The model under review builds one solid part; all positions refer to its coordinate system, in mm. A direction names the side the tool comes from. Give positions to 0.01 mm unless a question says otherwise; leave off trailing zeros. Loops run counter-clockwise (first coordinate to the right, second up) from the corner with the lowest first, then second, coordinate; pieces in that order, holes last. Notation, with made-up numbers: (-6, 11.25) - (10, 11.25) arc R20 cw to (10, 33.25) - close; hole circle Ø8 at (70.25, 88). An arc over 180 degrees is marked (long way). Return JSON: item names as keys, results as strings. Group by question number.
from build123d import *

# Parameters (mm, degrees)
SKETCH1_R               = 18
BOSS_EXTRUDE1_DEPTH     = 70
SKETCH2_R               = 2.5
BOSS_EXTRUDE2_DEPTH     = 17
CUT_EXTRUDE1_START      = -15
CUT_EXTRUDE1_DEPTH      = 15
SKETCH4_R               = 1.5875
CUT_EXTRUDE2_DEPTH      = 12.7
CIRPATTERN1_COUNT       = 6
BOSS_EXTRUDE3_START     = -2.032
BOSS_EXTRUDE3_DEPTH     = 8.382
BOSS_EXTRUDE4_DEPTH     = 12.0015
CUT_EXTRUDE3_REACH      = 99.88
CUT_EXTRUDE3_END_RADIUS = 18.8128
SKETCH7_R               = 2.159


with BuildPart() as part:
    # Sketch1 → Boss-Extrude1 (new body)
    with BuildSketch(Plane(origin=(0, 0, 0), x_dir=(1, 0, 0), z_dir=(0, 1, 0))):
        with Locations(Location((0, 0, 0), (0, 0, 270))):
            Circle(SKETCH1_R)
    extrude(amount=BOSS_EXTRUDE1_DEPTH)

    # Sketch2 → Boss-Extrude2 (add)
    with BuildSketch(Plane(origin=(0, 70, 0), x_dir=(1, 0, 0), z_dir=(0, 1, 0))):
        with Locations(Location((0, 0, 0), (0, 0, 270))):
            Circle(SKETCH2_R)
    extrude(amount=BOSS_EXTRUDE2_DEPTH)

    # Sketch3 → Cut-Extrude1 (cut)
    with BuildSketch(Plane(origin=(0, 87, 0), x_dir=(1, 0, 0), z_dir=(0, 1, 0)).offset(CUT_EXTRUDE1_START)):
        with BuildLine():
            Line((-1.5, 2), (1.5, 2))
            ThreePointArc((1.5, 2), (0, 2.5), (-1.5, 2))
        make_face()
    extrude(amount=CUT_EXTRUDE1_DEPTH, mode=Mode.SUBTRACT)

    # Sketch4 → Cut-Extrude2 (cut)
    with BuildSketch(Plane(origin=(0, 70, 0), x_dir=(1, 0, 0), z_dir=(0, 1, 0))):
        with Locations(Location((-6.25, 10.825317547, 0), (0, 0, 270))):
            Circle(SKETCH4_R)
    cut_extrude2 = extrude(amount=-CUT_EXTRUDE2_DEPTH, mode=Mode.SUBTRACT)

    # CirPattern1: Cut-Extrude2 ×6 about axis
    cirpattern1_axis = Axis((0, 0, 0), (0, 1, 0))
    for i in range(1, CIRPATTERN1_COUNT):
        add(cut_extrude2.rotate(cirpattern1_axis, i * 360 / CIRPATTERN1_COUNT), mode=Mode.SUBTRACT)

    # Sketch5 → Boss-Extrude3 (add)
    with BuildSketch(Plane.XZ.offset(BOSS_EXTRUDE3_START)):
        with BuildLine():
            Line((10.4775, -20.564736656), (10.4775, -14.636324462))
            ThreePointArc((10.4775, -14.636324462), (0, -18), (-10.4775, -14.636324462))
            Line((-10.4775, -14.636324462), (-10.4775, -20.564736656))
            ThreePointArc((-10.4775, -20.564736656), (0, -23.08), (10.4775, -20.564736656))
        make_face()
    extrude(amount=-BOSS_EXTRUDE3_DEPTH)

    # Sketch6 → Boss-Extrude4 (add)
    with BuildSketch(Plane.XZ):
        with BuildLine():
            Line((-11.2903, -14.018884617), (-11.2903, -15.048274644))
            ThreePointArc((-11.2903, -15.048274644), (0, -18.8128), (11.2903, -15.048274644))
            Line((11.2903, -15.048274644), (11.2903, -14.018884617))
            ThreePointArc((11.2903, -14.018884617), (0, -18), (-11.2903, -14.018884617))
        make_face()
    extrude(amount=-BOSS_EXTRUDE4_DEPTH)

    # Cut-Extrude3: up to this cylinder (the profile starts outside it)
    cut_extrude3_end = Plane(origin=(0, 6.223, 0), z_dir=(0, -1, 0)) * Cylinder(CUT_EXTRUDE3_END_RADIUS, 238.3856, mode=Mode.PRIVATE)
    # Sketch7 → Cut-Extrude3 (cut, up to the surface)
    with BuildSketch(Plane(origin=(0, 0, -23.08), x_dir=(-1, 0, 0), z_dir=(0, 0, -1)), mode=Mode.PRIVATE) as cut_extrude3_sk1:
        with Locations((-6.858, 6.223)):
            Circle(SKETCH7_R)
    cut_extrude3_tool1 = extrude(cut_extrude3_sk1.sketch, amount=-CUT_EXTRUDE3_REACH, mode=Mode.PRIVATE) - cut_extrude3_end
    add(cut_extrude3_tool1.solids().sort_by_distance((6.858, 6.223, -23.08))[0], mode=Mode.SUBTRACT)
    # Sketch7 → Cut-Extrude3 (cut, up to the surface)
    with BuildSketch(Plane(origin=(0, 0, -23.08), x_dir=(-1, 0, 0), z_dir=(0, 0, -1)), mode=Mode.PRIVATE) as cut_extrude3_sk2:
        with Locations((0, 6.223)):
            Circle(SKETCH7_R)
    cut_extrude3_tool2 = extrude(cut_extrude3_sk2.sketch, amount=-CUT_EXTRUDE3_REACH, mode=Mode.PRIVATE) - cut_extrude3_end
    add(cut_extrude3_tool2.solids().sort_by_distance((0, 6.223, -23.08))[0], mode=Mode.SUBTRACT)
    # Sketch7 → Cut-Extrude3 (cut, up to the surface)
    with BuildSketch(Plane(origin=(0, 0, -23.08), x_dir=(-1, 0, 0), z_dir=(0, 0, -1)), mode=Mode.PRIVATE) as cut_extrude3_sk3:
        with Locations((6.858, 6.223)):
            Circle(SKETCH7_R)
    cut_extrude3_tool3 = extrude(cut_extrude3_sk3.sketch, amount=-CUT_EXTRUDE3_REACH, mode=Mode.PRIVATE) - cut_extrude3_end
    add(cut_extrude3_tool3.solids().sort_by_distance((-6.858, 6.223, -23.08))[0], mode=Mode.SUBTRACT)


solid = part.part
Item 1: Tool access review of faces 4 (the face through (-6, 57.3, -11)), 5 (the face through (0, 2.032, -20)), 6 (the face through (0.468, 4.115, -20.915)), 7 (the face through (0, 10.414, -20)), 8 (the face through (-10.478, 6, -18)): name each direction out of +Z, -Z, +X, -X, +Y, -Y from which nothing blocks a thin tool from reaching the whole face with its end or side.
Item 2: Take a section at B-B (z = 11.5). State the section outline as (x, y) points.
Item 3: Take a section at D-D (x = -12.5). State the section outline as (y, z) points.
Item 4: Take a section at C-C (y = 35). State the section outline as (x, z) points.
Item 5: Take a section at A-A (x = 0). State the section outline as (y, z) points.
Item 6: For P1, Ø2.5, axis at x = 6.25, z = 10.83, coming from the +Y side; P2, Ø2, axis at x = -4, z = -18, coming from the +Y side; P3, Ø4, axis at y = 12, z = -14.5, coming from the +X side; P4, Ø2.5, axis at x = -6.25, z = 10.83, coming from the -Y side, all flat-tipped, find the tip position at first contact; note any pin that passes through.
Item 7: For L1, parallel to Y at x = 0, z = -22; L2, parallel to Y at x = -4, z = 12.5; L3, parallel to Y at x = 7, z = -10, list the stretches that pass through material, from the lowest coordinate up. Write a range as from..to.
Item 8: Mouldability with a two-part tool opening along Y and no side actions: class faces 1 (the face through (6, 57.3, -11)), 2 (the face through (-6.9, 6.2, -17.5)), 3 (the face through (10.95, 63.74, -0.34)) as +Y half, -Y half, draft (parallel to the pull), parting line (faces both ways), or undercut.
Check sheet entries:
{
 "1": {"face 4": "+Y", "face 5": "-Z, -Y", "face 6": "-Z", "face 7": "-Z, +Y", "face 8": "-Z, -X, +Y, -Y"},
 "2": {"outline": "(-13.85, 0) - (13.85, 0) - (13.85, 70) - (7.69, 70) - (7.69, 57.3) - (4.81, 57.3) - (4.81, 70) - (-4.81, 70) - (-4.81, 57.3) - (-7.69, 57.3) - (-7.69, 70) - (-13.85, 70) - close"},
 "3": {"outline": "(0, -12.95) - (70, -12.95) - (70, -1.59) - (57.3, -1.59) - (57.3, 1.59) - (70, 1.59) - (70, 12.95) - (0, 12.95) - close"},
 "4": {"outline": "circle Ø36 at (0, 0)"},
 "5": {"outline": "(0, -18.81) - (2.03, -18.81) - (2.03, -23.08) - (4.06, -23.08) - (4.06, -18.81) - (8.38, -18.81) - (8.38, -23.08) - (10.41, -23.08) - (10.41, -18.81) - (12, -18.81) - (12, -18) - (70, -18) - (70, -2.5) - (72, -2.5) - (72, -2) - (87, -2) - (87, 2.5) - (70, 2.5) - (70, 18) - (0, 18) - close"},
 "6": {"P1": "stops at y = 57.3", "P2": "stops at y = 70", "P3": "stops at x = 12.95", "P4": "stops at y = 0"},
 "7": {"L1": "y = 2.03..4.06, 8.38..10.41", "L2": "y = 0..70", "L3": "y = 0..57.3"},
 "8": {"face 1": "+Y half", "face 2": "undercut", "face 3": "draft"}
}
